```python
from build123d import *

# Parameters (mm, degrees)
F0_R            = 107.95
F1_DEPTH        = 12.7
F2_R            = 88.9
F3_DEPTH        = 203.2
F4_R            = 82.55
F5_DEPTH        = 203.2
F7_D            = 5.6134
F7_CSINK_D      = 10.4394
F7_CSINK_ANGLE  = 82
F7_COPIES_COUNT = 8


# Not quite as in the source:
# - a pattern or mirror of a feature is missing from the dataset's text; its kind, count and spacing are read off the source's solid


with BuildPart() as f1:
    # F0 (on Top) → F1 (new body)
    with BuildSketch(Plane.XY):
        Circle(F0_R)
    extrude(amount=-F1_DEPTH)

    # F2 (on face) → F3 (join)
    with BuildSketch(Plane(origin=(0, 0, -12.7), x_dir=(1, 0, 0), z_dir=(0, 0, -1))):
        Circle(F2_R)
    extrude(amount=F3_DEPTH)

    # F4 (on face) → F5 (cut)
    with BuildSketch(Plane.XY):
        Circle(F4_R)
    extrude(amount=-F5_DEPTH, mode=Mode.SUBTRACT)

    # F7 (through all)
    with Locations(Plane(origin=(0, 0, -12.7), x_dir=(1, 0, 0), z_dir=(0, 0, -1))):
        with Locations((0, -98.425)):
            f7 = CounterSinkHole(F7_D / 2, F7_CSINK_D / 2, counter_sink_angle=F7_CSINK_ANGLE)

    # F7_copies: F7 ×8 about axis
    f7_copies_axis = Axis((0, 0, 0), (0, 0, 1))
    for i in range(1, F7_COPIES_COUNT):
        add(f7.rotate(f7_copies_axis, i * 360 / F7_COPIES_COUNT), mode=Mode.SUBTRACT)


solid = f1.part
```
Work out the finished part from the listing and answer in its coordinate system (mm). A direction names the side the tool comes from. Give positions to 0.01 mm unless a question says otherwise; leave off trailing zeros. Loops run counter-clockwise (first coordinate to the right, second up) from the corner with the lowest first, then second, coordinate; pieces in that order, holes last. Notation, with made-up numbers: (-3, 86) -> (46, 86) arc R27 ccw to (46, 115) -> close; hole circle Ø4 at (13.5, 29.25). An arc over 180 degrees is marked (long way). One line per question, with ' | ' between items. Start each with the question number.
1) Section B-B, the plane z = -48 is taken. Determine the outline of the cut face in (x, y), then the cut area to 3 significant figures.
2) Section C-C, the plane y = 48 is taken. Determine the outline of the cut face in (x, z).
3) Each of these flat-tipped pins is pushed along its axis until it touches: pin 1 (12 mm diameter, centred on y = -45.5, z = -99.5, fed in from -X); pin 2 (6 mm diameter, centred on x = -82.5, z = -42, fed in from -Y); pin 3 (3 mm diameter, centred on y = -72, z = -28, fed in from -X). Where does it stop, or does it pass through?
4) Section A-A, the plane x = 34 is taken. Determine the outline of the cut face in (y, z), then the cut area to 3 significant figures.
5) Straight lines are drawn through the part: L1, parallel to Y at x = 0, z = -5; L2, parallel to X at y = -1, z = -120; L3, parallel to Z at x = 9.5, y = -81. For each, find the intervals that lie inside material, in ascending order.
6) Determine the mould class of faces 1 (the face through (-79.56, 72.96, -6.26)), 2 (the face through (-24.5, -79.5, 0)), 3 (the face through (100.204, -2.32, -10.059)) for opening direction X: +X half, -X half, draft (parallel to the pull), parting line (faces both ways), or undercut.
7) For faces 4 (the face through (-1, 1, -203.2)), 5 (the face through (-72.38, -69.23, -4.89)), determine the directions among +Z, -Z, +X, -X, +Y, -Y from which every point of the face is accessible in a straight line to the end or side of a thin tool.
Resolved:
1) outline: circle Ø177.8 at (0, 0); hole circle Ø165.1 at (0, 0) | area: 3,420 mm2
2) outline: (-96.69, -12.7) -> (-74.83, -12.7) -> (-74.83, -215.9) -> (74.83, -215.9) -> (74.83, -12.7) -> (96.69, -12.7) -> (96.69, 0) -> (67.16, 0) -> (67.16, -203.2) -> (-67.16, -203.2) -> (-67.16, 0) -> (-96.69, 0) -> close
3) pin 1: x = -79.64 | pin 2: y = -39.79 | pin 3: x = -54.16
4) outline: (-102.46, -12.7) -> (-82.14, -12.7) -> (-82.14, -215.9) -> (82.14, -215.9) -> (82.14, -12.7) -> (102.46, -12.7) -> (102.46, 0) -> (75.22, 0) -> (75.22, -203.2) -> (-75.22, -203.2) -> (-75.22, 0) -> (-102.46, 0) -> close | area: 5,410 mm2
5) L1: -107.95 to -101.23, -95.62 to -82.55, 82.55 to 95.62, 101.23 to 107.95 | L2: -88.89 to -82.54, 82.54 to 88.89 | L3: -215.9 to -203.2
6) face 1: parting line | face 2: draft | face 3: undercut
7) face 4: +Z | face 5: +Z, -Z
